Autodesk Inventor part; units mm, degrees
ref_plane "YZ Plane" through (0, 0, 0) normal (1, 0, 0) x (0, 1, 0)
ref_plane "XZ Plane" through (0, 0, 0) normal (0, 1, 0) x (-1, 0, 0)
ref_plane "XY Plane" through (0, 0, 0) normal (0, 0, 1) x (1, 0, 0)
sketch "Sketch1" plane through (0, 0, 0) normal (0, 0, 1) x (1, 0, 0)
  circle A0 centre (0, 0) radius 5
  circle A1 centre (0, 0) radius 2.5
  dimension "d0" = 10
  dimension "d1" = 5
extrude "Extrusion1" add sketch "Sketch1" along normal blind 116 contours A0 | A1
extrude "Extrusion2" add sketch "Sketch1" along normal blind 44 from surface at 116 contours A1
extrude "Extrusion3" add sketch "Sketch1" against normal blind 44 contours A1
properties part number "Main Shaft"
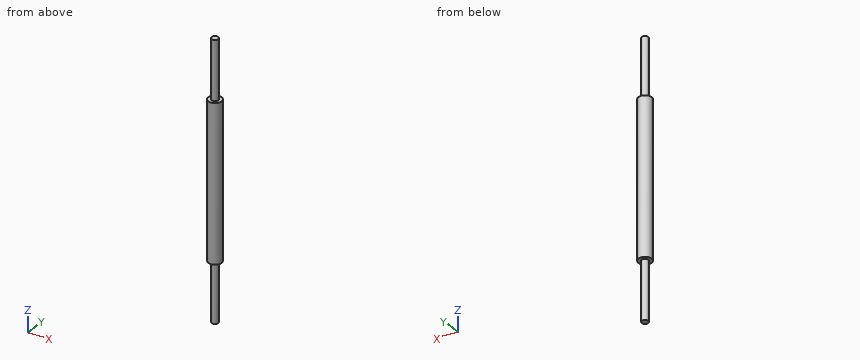
Read the model definition and answer for the solid it produces. Units are mm, in the model's axes. Give positions to 0.01 mm unless a question says otherwise; leave off trailing zeros. Write each loop counter-clockwise with the first axis right and the second up, starting at its lowest first coordinate (ties: lowest second). Pieces come first, ordered by that corner, then holes. Notation, with made-up numbers: (-22, 51) -> (4, 51) arc R11 cw to (4, 59) -> close; hole circle Ø11 at (53, -30.5). An arc over 180 degrees is marked (long way). Answer as a JSON object with one key per item and string values. Group by question number.
1) Consider L1, parallel to Z at x = 2.75, y = -1; L2, parallel to X at y = -0.25, z = 115; L3, parallel to X at y = -4.25, z = 16. Determine where each line is inside the solid, lowest interval first. Write a range as from..to.
2) Find section A-A (x = 0). Write down the section's boundary in (y, z), and give its area (3 significant figures).
3) Each of these flat-tipped pins is pushed along its axis until it touches: P1, Ø3, axis at y = -2.5, z = 121, coming from the -X side; P2, Ø2, axis at y = -2.5, z = 5, coming from the -X side. Where does it stop, or does it pass through?
4) Find section C-C (z = -25). Write down the section's boundary in (x, y).
Values follow:
{
 "1": {"L1": "z = 0..116", "L2": "x = -4.99..4.99", "L3": "x = -2.63..2.63"},
 "2": {"outline": "(-5, 0) -> (-2.5, 0) -> (-2.5, -44) -> (2.5, -44) -> (2.5, 0) -> (5, 0) -> (5, 116) -> (2.5, 116) -> (2.5, 160) -> (-2.5, 160) -> (-2.5, 116) -> (-5, 116) -> close", "area": "1,600 mm2"},
 "3": {"P1": "stops at x = -2.29", "P2": "stops at x = -4.77"},
 "4": {"outline": "circle Ø5 at (0, 0)"}
}
